For this review, take the finished solid that the model builds, in its own axes (mm). A direction names the side the tool comes from. Round coordinates to 2 decimals unless told otherwise and drop trailing zeros. Loops run counter-clockwise (first coordinate to the right, second up) from the corner with the lowest first, then second, coordinate; pieces in that order, holes last. Notation, with made-up numbers: (83, 33) -> (118, 33) arc R16 cw to (118, 43) -> close; hole circle Ø6 at (72.5, -1). An arc over 180 degrees is marked (long way). One line per question, with ' | ' between items. Start each with the question number.
1. For pin 1 Ø1.5 at (x, z) = (1, 2) entering from -Y; pin 2 Ø1 at (y, z) = (-1.5, 2) entering from -X, all flat-tipped, find the tip position at first contact; note any pin that passes through.
2. Wall thickness on line 1 along Y through (x, z) = (0, 2.75); line 2 along Y through (x, z) = (0.75, 4.25); line 3 along X through (y, z) = (0.9, 2.75): over which ranges is each line inside the solid? List them lowest first.
3. Consider section A-A (x = 0). Write out the cut boundary in (y, z), and give its area (4 significant figures).
4. Draft analysis for pull direction X (two halves, no side actions). For faces 3 (the face through (0, 1, 3)), 4 (the face through (0, -2, 4)), 5 (the face through (1, -1, 0)), state which applies: pulls with the +X half, pulls with the -X half, needs draft (parallel to the pull), parting line crosses it, or undercut.
5. Consider section C-C (z = 4.25). Write out the cut boundary in (x, y), and give its area (3 significant figures).
6. For faces 1 (the face through (0, 0, 7)), 2 (the face through (0, 0, 8)), list the 3-axis set-ups (+Z, -Z, +X, -X, +Y, -Y) from which the entire face can be reached by the end or side of a thin tool; tool diameter is ignored.
```python
from build123d import *

# Parameters (mm, degrees)
F0_R     = 2
F1_DEPTH = 8
F2_R     = 1
F3_DEPTH = 7
F4_SIZE  = 0.5


with BuildPart() as f1:
    # F0 (on Top) → F1 (new body)
    with BuildSketch(Plane.XY):
        Circle(F0_R)
    extrude(amount=F1_DEPTH)

    # F2 (on face) → F3 (cut)
    with BuildSketch(Plane(origin=(0, 0, 0), x_dir=(1, 0, 0), z_dir=(0, 0, -1))):
        Circle(F2_R)
    extrude(amount=-F3_DEPTH, mode=Mode.SUBTRACT)

    # F4
    f4_edges = [f1.edges().sort_by_distance(p)[0] for p in [
        (-2, 0, 8),
    ]]
    chamfer(f4_edges, length=F4_SIZE)


solid = f1.part
```
Answer block:
1) pin 1: stops at y = -1.98 | pin 2: stops at x = -1.73
2) line 1: y = -2 to -1, 1 to 2 | line 2: y = -1.85 to -0.66, 0.66 to 1.85 | line 3: x = -1.79 to -0.44, 0.44 to 1.79
3) outline: (-2, 0) -> (-1, 0) -> (-1, 7) -> (1, 7) -> (1, 0) -> (2, 0) -> (2, 7.5) -> (1.5, 8) -> (-1.5, 8) -> (-2, 7.5) -> close | area: 17.75 mm2
4) face 3: undercut | face 4: parting line crosses it | face 5: needs draft
5) outline: circle Ø4 at (0, 0); hole circle Ø2 at (0, 0) | area: 9.42 mm2
6) face 1: -Z | face 2: +Z, +X, -X, +Y, -Y
